The model under review builds one solid part; all positions refer to its coordinate system, in mm. Give positions to 0.01 mm unless a question says otherwise; leave off trailing zeros. Write each loop counter-clockwise with the first axis right and the second up, starting at its lowest first coordinate (ties: lowest second). Pieces come first, ordered by that corner, then holes.
from build123d import *

# Parameters (mm, degrees)
SKETCH_1_W                        = 1541
SKETCH_1_H                        = 151
SM_BASE_FLANGE_1_DEPTH            = 1
SM_EDGE_FLANGE_1_STRIP_W          = 5.4732
SM_EDGE_FLANGE_1_STRIP_H          = 1
SM_EDGE_FLANGE_1_STRIP_CUT_DEPTH  = 1441
SM_EDGE_FLANGE_1_RELIEF_W         = 5.9732
SM_EDGE_FLANGE_1_RELIEF_H         = 0.5
SM_EDGE_FLANGE_1_RELIEF_CUT_DEPTH = 1
SM_EDGE_FLANGE_1_DEPTH            = 1441
SM_EDGE_FLANGE_2_STRIP_W          = 5.4732
SM_EDGE_FLANGE_2_STRIP_H          = 1
SM_EDGE_FLANGE_2_STRIP_CUT_DEPTH  = 1441
SM_EDGE_FLANGE_2_RELIEF_W         = 5.9732
SM_EDGE_FLANGE_2_RELIEF_H         = 0.5
SM_EDGE_FLANGE_2_RELIEF_CUT_DEPTH = 1
SM_EDGE_FLANGE_2_DEPTH            = 1441
SM_EDGE_FLANGE_3_STRIP_W          = 5.4732
SM_EDGE_FLANGE_3_STRIP_H          = 1
SM_EDGE_FLANGE_3_STRIP_CUT_DEPTH  = 51
SM_EDGE_FLANGE_3_RELIEF_W         = 5.9732
SM_EDGE_FLANGE_3_RELIEF_H         = 0.5
SM_EDGE_FLANGE_3_RELIEF_CUT_DEPTH = 1
SM_EDGE_FLANGE_3_DEPTH            = 51
SM_EDGE_FLANGE_4_STRIP_W          = 5.4732
SM_EDGE_FLANGE_4_STRIP_H          = 1
SM_EDGE_FLANGE_4_STRIP_CUT_DEPTH  = 51
SM_EDGE_FLANGE_4_RELIEF_W         = 5.9732
SM_EDGE_FLANGE_4_RELIEF_H         = 0.5
SM_EDGE_FLANGE_4_RELIEF_CUT_DEPTH = 1
SM_EDGE_FLANGE_4_DEPTH            = 51
SKETCH_15_R                       = 3
CUT_EXTRUDE_1_DEPTH               = 775.44851346


# Sheet-metal steps are written as plain solids
with BuildPart() as part:
    # Sketch 1 → 基体-法兰1 (new body)
    with BuildSketch(Plane.XY):
        Rectangle(SKETCH_1_W, SKETCH_1_H)
    extrude(amount=-SM_BASE_FLANGE_1_DEPTH)

    # 边线-法兰1 strip (across the edge) → 边线-法兰1 strip cut (cut)
    with BuildSketch(Plane(origin=(-720.5, 75.5, -1), x_dir=(0, -1, 0), z_dir=(1, 0, 0))):
        with Locations((-1, -0.5)):
            Rectangle(SM_EDGE_FLANGE_1_STRIP_W, SM_EDGE_FLANGE_1_STRIP_H)
    extrude(amount=SM_EDGE_FLANGE_1_STRIP_CUT_DEPTH, mode=Mode.SUBTRACT)

    # 边线-法兰1 relief (on the sheet) → 边线-法兰1 relief cut (cut)
    with BuildSketch(Plane(origin=(-720.5, 73.7634, -1), x_dir=(0, -1, 0), z_dir=(0, 0, -1))):
        with Locations((-2.4866, 0.25)):
            Rectangle(SM_EDGE_FLANGE_1_RELIEF_W, SM_EDGE_FLANGE_1_RELIEF_H)
        with Locations((-2.4866, -1441.25)):
            Rectangle(SM_EDGE_FLANGE_1_RELIEF_W, SM_EDGE_FLANGE_1_RELIEF_H)
    extrude(amount=-SM_EDGE_FLANGE_1_RELIEF_CUT_DEPTH, mode=Mode.SUBTRACT)

    # 边线-法兰1 section (across the edge) → 边线-法兰1 (add)
    with BuildSketch(Plane(origin=(-720.5, 75.5, -1), x_dir=(0, -1, 0), z_dir=(1, 0, 0))):
        with BuildLine():
            Line((0, 0.7366), (0, 19))
            Line((0, 19), (1, 19))
            Line((1, 19), (1, 0.7366))
            ThreePointArc((1, 0.7366), (1.215745145, 0.215745145), (1.7366, 0))
            Line((1.7366, 0), (1.7366, -1))
            ThreePointArc((1.7366, -1), (0.508638364, -0.491361636), (0, 0.7366))
        make_face()
    extrude(amount=SM_EDGE_FLANGE_1_DEPTH)

    # 边线-法兰2 strip (across the edge) → 边线-法兰2 strip cut (cut)
    with BuildSketch(Plane(origin=(720.5, -75.5, -1), x_dir=(0, 1, 0), z_dir=(-1, 0, 0))):
        with Locations((-1, -0.5)):
            Rectangle(SM_EDGE_FLANGE_2_STRIP_W, SM_EDGE_FLANGE_2_STRIP_H)
    extrude(amount=SM_EDGE_FLANGE_2_STRIP_CUT_DEPTH, mode=Mode.SUBTRACT)

    # 边线-法兰2 relief (on the sheet) → 边线-法兰2 relief cut (cut)
    with BuildSketch(Plane(origin=(720.5, -73.7634, -1), x_dir=(0, 1, 0), z_dir=(0, 0, -1))):
        with Locations((-2.4866, 0.25)):
            Rectangle(SM_EDGE_FLANGE_2_RELIEF_W, SM_EDGE_FLANGE_2_RELIEF_H)
        with Locations((-2.4866, -1441.25)):
            Rectangle(SM_EDGE_FLANGE_2_RELIEF_W, SM_EDGE_FLANGE_2_RELIEF_H)
    extrude(amount=-SM_EDGE_FLANGE_2_RELIEF_CUT_DEPTH, mode=Mode.SUBTRACT)

    # 边线-法兰2 section (across the edge) → 边线-法兰2 (add)
    with BuildSketch(Plane(origin=(720.5, -75.5, -1), x_dir=(0, 1, 0), z_dir=(-1, 0, 0))):
        with BuildLine():
            Line((0, 0.7366), (0, 19))
            Line((0, 19), (1, 19))
            Line((1, 19), (1, 0.7366))
            ThreePointArc((1, 0.7366), (1.215745145, 0.215745145), (1.7366, 0))
            Line((1.7366, 0), (1.7366, -1))
            ThreePointArc((1.7366, -1), (0.508638364, -0.491361636), (0, 0.7366))
        make_face()
    extrude(amount=SM_EDGE_FLANGE_2_DEPTH)

    # 边线-法兰3 strip (across the edge) → 边线-法兰3 strip cut (cut)
    with BuildSketch(Plane(origin=(770.5, 25.5, -1), x_dir=(-1, 0, 0), z_dir=(0, -1, 0))):
        with Locations((-1, -0.5)):
            Rectangle(SM_EDGE_FLANGE_3_STRIP_W, SM_EDGE_FLANGE_3_STRIP_H)
    extrude(amount=SM_EDGE_FLANGE_3_STRIP_CUT_DEPTH, mode=Mode.SUBTRACT)

    # 边线-法兰3 relief (on the sheet) → 边线-法兰3 relief cut (cut)
    with BuildSketch(Plane(origin=(768.7634, 25.5, -1), x_dir=(-1, 0, 0), z_dir=(0, 0, -1))):
        with Locations((-2.4866, 0.25)):
            Rectangle(SM_EDGE_FLANGE_3_RELIEF_W, SM_EDGE_FLANGE_3_RELIEF_H)
        with Locations((-2.4866, -51.25)):
            Rectangle(SM_EDGE_FLANGE_3_RELIEF_W, SM_EDGE_FLANGE_3_RELIEF_H)
    extrude(amount=-SM_EDGE_FLANGE_3_RELIEF_CUT_DEPTH, mode=Mode.SUBTRACT)

    # 边线-法兰3 section (across the edge) → 边线-法兰3 (add)
    with BuildSketch(Plane(origin=(770.5, 25.5, -1), x_dir=(-1, 0, 0), z_dir=(0, -1, 0))):
        with BuildLine():
            Line((0, 0.7366), (0, 19))
            Line((0, 19), (1, 19))
            Line((1, 19), (1, 0.7366))
            ThreePointArc((1, 0.7366), (1.215745145, 0.215745145), (1.7366, 0))
            Line((1.7366, 0), (1.7366, -1))
            ThreePointArc((1.7366, -1), (0.508638364, -0.491361636), (0, 0.7366))
        make_face()
    extrude(amount=SM_EDGE_FLANGE_3_DEPTH)

    # 边线-法兰4 strip (across the edge) → 边线-法兰4 strip cut (cut)
    with BuildSketch(Plane(origin=(-770.5, -25.5, -1), x_dir=(1, 0, 0), z_dir=(0, 1, 0))):
        with Locations((-1, -0.5)):
            Rectangle(SM_EDGE_FLANGE_4_STRIP_W, SM_EDGE_FLANGE_4_STRIP_H)
    extrude(amount=SM_EDGE_FLANGE_4_STRIP_CUT_DEPTH, mode=Mode.SUBTRACT)

    # 边线-法兰4 relief (on the sheet) → 边线-法兰4 relief cut (cut)
    with BuildSketch(Plane(origin=(-768.7634, -25.5, -1), x_dir=(1, 0, 0), z_dir=(0, 0, -1))):
        with Locations((-2.4866, 0.25)):
            Rectangle(SM_EDGE_FLANGE_4_RELIEF_W, SM_EDGE_FLANGE_4_RELIEF_H)
        with Locations((-2.4866, -51.25)):
            Rectangle(SM_EDGE_FLANGE_4_RELIEF_W, SM_EDGE_FLANGE_4_RELIEF_H)
    extrude(amount=-SM_EDGE_FLANGE_4_RELIEF_CUT_DEPTH, mode=Mode.SUBTRACT)

    # 边线-法兰4 section (across the edge) → 边线-法兰4 (add)
    with BuildSketch(Plane(origin=(-770.5, -25.5, -1), x_dir=(1, 0, 0), z_dir=(0, 1, 0))):
        with BuildLine():
            Line((0, 0.7366), (0, 19))
            Line((0, 19), (1, 19))
            Line((1, 19), (1, 0.7366))
            ThreePointArc((1, 0.7366), (1.215745145, 0.215745145), (1.7366, 0))
            Line((1.7366, 0), (1.7366, -1))
            ThreePointArc((1.7366, -1), (0.508638364, -0.491361636), (0, 0.7366))
        make_face()
    extrude(amount=SM_EDGE_FLANGE_4_DEPTH)

    # 草图15 → 切除-拉伸1 (cut, through all)
    with BuildSketch(Plane.XY):
        with Locations((761, 66)):
            Circle(SKETCH_15_R)
        with Locations((761, -66)):
            Circle(SKETCH_15_R)
        with Locations((-761, 66)):
            Circle(SKETCH_15_R)
        with Locations((-761, -66)):
            Circle(SKETCH_15_R)
    extrude(amount=-CUT_EXTRUDE_1_DEPTH, mode=Mode.SUBTRACT)


solid = part.part
1) Consider section A-A, the plane z = -9.5. Give the boundary of the cut face in (x, y), then the cut area to 3 significant figures.
2) The part is to be moulded in two halves that separate along X. For faces 1 (the flat face through (-11, 1, -1)), 2 (the flat face through (-11, 1, 0)), say which applies: +X half, -X half, draft (parallel to the pull), parting line (faces both ways), or undercut.
3) Consider section C-C, the plane y = -7. Give the boundary of the cut face in (x, z).
4) Insertion check: pin 1 (3 mm diameter, centred on x = 368, y = -53, fed in from -Z); pin 2 (0.7 mm diameter, centred on x = 769, z = -12, fed in from +Y); pin 3 (1.1 mm diameter, centred on y = 74.5, z = -12.5, fed in from -X); pin 4 (1.8 mm diameter, centred on x = -769, z = -12.5, fed in from -Y). Each pin has a flat end and moves straight along its axis. Give the tip position at first contact, or say it passes through.
5) Consider section B-B, the plane x = -95.5. Give the boundary of the cut face in (y, z).
6) To check wall thickness, follow probe 1 along Y at (x, z) = (761, -0.8); probe 2 along X at (y, z) = (-21.5, -8.25); probe 3 along Y at (x, z) = (-457.5, -5.5). State the ranges of each line that lie inside material, in increasing order.
Answer block:
1. outline: (-770.5, -25.5) - (-769.5, -25.5) - (-769.5, 25.5) - (-770.5, 25.5) - close; (-720.5, -75.5) - (720.5, -75.5) - (720.5, -74.5) - (-720.5, -74.5) - close; (-720.5, 74.5) - (720.5, 74.5) - (720.5, 75.5) - (-720.5, 75.5) - close; (769.5, -25.5) - (770.5, -25.5) - (770.5, 25.5) - (769.5, 25.5) - close
1. area: 2,980 mm2
2. face 1: undercut
2. face 2: draft
3. outline: (-770.5, -20) - (-769.5, -20) - (-769.5, -1.74) arc R0.74 cw to (-768.76, -1) - (768.76, -1) arc R0.74 cw to (769.5, -1.74) - (769.5, -20) - (770.5, -20) - (770.5, -1.74) arc R1.74 ccw to (768.76, 0) - (-768.76, 0) arc R1.74 ccw to (-770.5, -1.74) - close
4. pin 1: stops at z = -1
4. pin 2: passes through
4. pin 3: stops at x = -720.5
4. pin 4: stops at y = -25.5
5. outline: (-75.5, -20) - (-74.5, -20) - (-74.5, -1.74) arc R0.74 cw to (-73.76, -1) - (73.76, -1) arc R0.74 cw to (74.5, -1.74) - (74.5, -20) - (75.5, -20) - (75.5, -1.74) arc R1.74 ccw to (73.76, 0) - (-73.76, 0) arc R1.74 ccw to (-75.5, -1.74) - close
6. probe 1: y = -75.5 to -69, -63 to 63, 69 to 75.5
6. probe 2: x = -770.5 to -769.5, 769.5 to 770.5
6. probe 3: y = -75.5 to -74.5, 74.5 to 75.5
